Model file for the job. Use its own axes, mm. Face numbers are marked on the shaded views. A direction names the side the tool comes from. Give positions to 0.01 mm unless a question says otherwise; leave off trailing zeros. Write each loop counter-clockwise with the first axis right and the second up, starting at its lowest first coordinate (ties: lowest second). Pieces come first, ordered by that corner, then holes.
```python
from build123d import *

# Parameters (mm, degrees)
F0_W     = 1117.6
F0_H     = 685.8
F1_DEPTH = 25.4
F2_W     = 387.35
F2_H     = 489.712
F3_DEPTH = 292.1
F5_DEPTH = 317.5


with BuildPart() as f1:
    # F0 (on Top) → F1 (new body)
    with BuildSketch(Plane.XY):
        Rectangle(F0_W, F0_H)
    extrude(amount=-F1_DEPTH)

    # F2 (on face) → F3 (join)
    with BuildSketch(Plane(origin=(0, 0, -25.4), x_dir=(1, 0, 0), z_dir=(0, 0, -1))):
        with Locations((0, -98.044)):
            Rectangle(F2_W, F2_H)
    extrude(amount=F3_DEPTH)

    # F4 (on face) → F5 (join)
    with BuildSketch(Plane(origin=(-193.675, 0, 0), x_dir=(0, -1, 0), z_dir=(-1, 0, 0))):
        with BuildLine():
            Line((-342.9, -105.342755), (-597.796015, -173.641936))
            ThreePointArc((-597.796015, -173.641936), (-650.314815, -335.895403), (-480.768299, -317.5))
            Line((-480.768299, -317.5), (-342.9, -317.5))
            Line((-342.9, -317.5), (-342.9, -105.342755))
        make_face()
    extrude(amount=-F5_DEPTH)


solid = f1.part
```
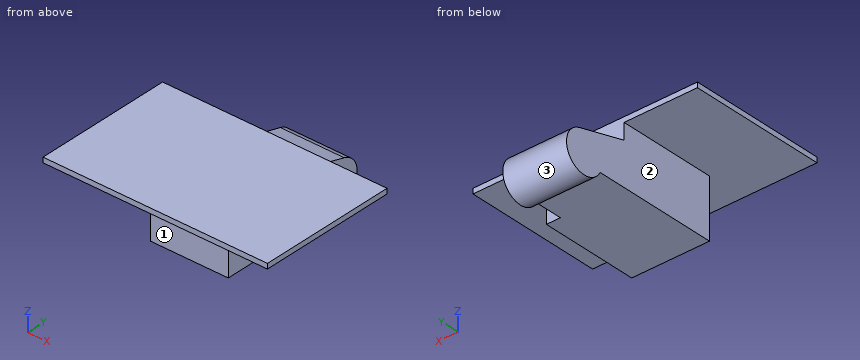
1. Slice it at B-B, the plane y = 107. Write the cut outline in (x, z) (3 decimals), and give its area (3 significant figures).
Calculated:
outline: (-558.8, -25.4) - (-193.675, -25.4) - (-193.675, -317.5) - (193.675, -317.5) - (193.675, -25.4) - (558.8, -25.4) - (558.8, 0) - (-558.8, 0) - close
area: 142,000 mm2
2. Which spindle directions (+Z, -Z, +X, -X, +Y, -Y) get a long thin tool onto all of the face, cutting with end or side? Do the marked faces 1, 2 and 3. Say none if no direction does.
Calculated:
face 1: -Z, +X, -X, -Y
face 2: -Z, -X, +Y, -Y
face 3: +X, -X
3. Slice it at C-C, the plane z = -271.78. Write the cut outline in (x, y) (3 decimals), and give its area (3 significant figures).
Calculated:
outline: (-193.675, -146.812) - (193.675, -146.812) - (193.675, 342.9) - (123.825, 342.9) - (123.825, 673.1) - (-193.675, 673.1) - close
area: 295,000 mm2
4. Probe probe 1 along Z at (x, y) = (-387, 27); probe 2 along Z at (x, y) = (-178.5, 13); probe 3 along X at (y, z) = (193, -110.5) (3 decimals). List the from-to ranges inside material, lowest first.
Calculated:
probe 1: z = -25.4 to 0
probe 2: z = -317.5 to 0
probe 3: x = -193.675 to 193.675
5. Slice it at A-A, the plane x = -134. Write the cut outline in (y, z).
Calculated:
outline: (-342.9, -25.4) - (-146.81, -25.4) - (-146.81, -317.5) - (480.77, -317.5) arc R101.6 ccw (long way) to (597.8, -173.64) - (342.9, -105.34) - (342.9, 0) - (-342.9, 0) - close
6. Slice it at D-D, the plane z = -43. Write the cut outline in (x, y) (3 decimals).
Calculated:
outline: (-193.675, -146.812) - (193.675, -146.812) - (193.675, 342.9) - (-193.675, 342.9) - close
7. Pin check, flat tips, straight feed: P1, Ø3, axis at x = -92.5, z = -221.5, coming from the +Y side; P2, Ø2, axis at x = 95.5, z = -136, coming from the -Y side; P3, Ø1, axis at x = -163.5, z = -306, coming from the +Y side. Stop position of each tip, or through.
Calculated:
P1: stops at y = 660.62
P2: stops at y = -146.81
P3: stops at y = 667.34
